The model under review builds one solid part; all positions refer to its coordinate system, in mm. A direction names the side the tool comes from. Coordinates: 2 decimals unless noted, no trailing zeros. Loops run counter-clockwise (first coordinate to the right, second up) from the corner with the lowest first, then second, coordinate; pieces in that order, holes last. Notation, with made-up numbers: (-4.75, 40) - (15.25, 40) arc R38 ccw to (15.25, 79) - close; hole circle Ø4 at (-37, 46.5). An arc over 180 degrees is marked (long way). One line per item, written item: value. Start each with the question number.
1. Insertion check: P1, Ø1.9, axis at x = 9, z = 8.5, coming from the -Y side; P2, Ø4, axis at x = 19.5, z = 2, coming from the +Y side; P3, Ø1.5, axis at x = 28, z = 8.5, coming from the +Y side. Each pin has a flat end and moves straight along its axis. Give the tip position at first contact, or say it passes through.
2. We need section B-B, the plane y = 3.5. Give the boundary of the cut face in (x, z), then the cut area to 3 significant figures.
3. We need section C-C, the plane x = 32. Give the boundary of the cut face in (y, z), then the cut area to 3 significant figures.
4. Mouldability with a two-part tool opening along X and no side actions: class faces 1 (the face through (29.115, -11.529, 7.395)), 2 (the face through (6.298, -2.507, 7.395)), 3 (the face through (14, 6, 15)), 4 (the face through (8.047, 13.33, 7.395)) as +X half, -X half, draft (parallel to the pull), parting line (faces both ways), or undercut.
5. For faces 5 (the face through (8.59, 13.79, 7.61)), 6 (the face through (16, 23, 7)), 7 (the face through (8, 23, 8)), 8 (the face through (5.8, 23.74, 7.53)), list the 3-axis set-ups (+Z, -Z, +X, -X, +Y, -Y) from which the entire face can be reached by the end or side of a thin tool; tool diameter is ignored.
6. To check wall thickness, follow line 1 (X direction, y = 0, z = 11); line 2 (X direction, y = -5, z = 13); line 3 (Y direction, x = 23, z = 2.5). State the ranges of each line that lie inside material, in increasing order.
from build123d import *

# Parameters (mm, degrees)
F1_DEPTH      = 15
F4_DEPTH      = 9.2
F4_DEPTH_BACK = 1
F7_DEPTH      = 1.5
F8_SIZE       = 1.49999
F9_R          = 5
F11_DEPTH     = 4
F12_T4_DEPTH  = 6.4753623201
F12_S5_R      = 22.299103121
F12_T6_DEPTH  = 5
F12_S8_R      = 5
F12_T9_DEPTH  = 5
F12_T13_DEPTH = 6.4753623415
F12_S15_R     = 5
F12_T16_DEPTH = 5
F12_S17_R     = 22.299103121
F12_T18_DEPTH = 5


# Not quite as in the source:
# - a fillet or chamfer that OpenCascade refuses, or shapes differently, is made with other operations: its cross-section is extruded or revolved along the edge and cut away or added
# - a fillet or chamfer is up to 0.001 mm smaller than in the source, because OpenCascade refuses the exact size


with BuildPart() as f1:
    # F0 (on Top) → F1 (new body)
    with BuildSketch(Plane.XY):
        with BuildLine():
            Line((37.0060966544, -19.4203102168), (21, -3.4142135624))
            Line((21, -3.4142135624), (21, 23))
            Line((21, 23), (8.9, 23))
            Line((8.9, 23), (8.0008047996, 12.8091210619))
            ThreePointArc((8.0008047996, 12.8091210619), (7.9975966714, 12.8026247244), (7.9908435011, 12.8))
            Line((7.9908435011, 12.8), (6.1708946074, 12.8))
            ThreePointArc((6.1708946074, 12.8), (3.6860466407, 11.9345702389), (2.2764293651, 9.7127652912))
            Line((2.2764293651, 9.7127652912), (-0.46875, -2))
            Line((-0.46875, -2), (-4.7960747033, -3))
            Line((-4.7960747033, -3), (17.7071067812, -2))
            Line((17.7071067812, -2), (17.7071067812, -4.7781745931))
            Line((17.7071067812, -4.7781745931), (34.6776695297, -21.7487373415))
            Line((34.6776695297, -21.7487373415), (37.0060966544, -19.4203102168))
        make_face()
    extrude(amount=F1_DEPTH)

    # F3 (on face) → F4 (cut, two sides)
    with BuildSketch(Plane(origin=(2.0824892704, 23.6015450644, 0), x_dir=(0.99612985, -0.0878938103, 0), z_dir=(-0.0878938103, -0.99612985, 0))) as f4_sk:
        with BuildLine():
            Line((6.8439980284, 15), (6.8439980284, 0))
            ThreePointArc((6.8439980284, 0), (8.1431011494, 7.5), (6.8439980284, 15))
        make_face()
    extrude(amount=F4_DEPTH, mode=Mode.SUBTRACT)
    extrude(f4_sk.sketch, amount=-F4_DEPTH_BACK, mode=Mode.SUBTRACT)

    # F6 (on offset) → F7 (join)
    with BuildSketch(Plane(origin=(0, 23, 0), x_dir=(-1, 0, 0), z_dir=(0, 1, 0))):
        with BuildLine():
            ThreePointArc((-7.0033527857, 9.4235612132), (-7.0960699027, 7.4999998768), (-7.0033527857, 5.5764385404))
            Line((-7.0033527857, 5.5764385404), (-5.4957957644, 5.5764385404))
            ThreePointArc((-5.4957957644, 5.5764385404), (-5.5960699027, 7.4999998768), (-5.4957957644, 9.4235612132))
            Line((-5.4957957644, 9.4235612132), (-7.0033527857, 9.4235612132))
        make_face()
        with BuildLine():
            Line((-14.0960699027, 7.4999998768), (-14.0960699027, 5.5764385404))
            Line((-14.0960699027, 5.5764385404), (-7.0033527857, 5.5764385404))
            ThreePointArc((-7.0033527857, 5.5764385404), (-7.0960699027, 7.4999998768), (-7.0033527857, 9.4235612132))
            Line((-7.0033527857, 9.4235612132), (-14.0960699027, 9.4235612132))
            Line((-14.0960699027, 9.4235612132), (-14.0960699027, 7.4999998768))
        make_face()
    extrude(amount=F7_DEPTH)

    # F8 (size 1.5 in the source; OpenCascade refuses exactly that, so slightly less here)
    f8_edges = [f1.edges().sort_by_distance(p)[0] for p in [
        (14.09607, 24.5, 7.5),
    ]]
    chamfer(f8_edges, length=F8_SIZE)

    # F9
    f9_edges = [f1.edges().sort_by_distance(p)[0] for p in [
        (12.59608, 24.5, 7.5),
    ]]
    fillet(f9_edges, radius=F9_R)

    # F10 (on face) → F11 (cut)
    with BuildSketch(Plane.XY.offset(9.4235612132)):
        Polygon((5.4957957644, 22), (6.5002299745, 22), (5.4957957644, 24.5), align=None)
    extrude(amount=-F11_DEPTH, mode=Mode.SUBTRACT)

    # F12: fillet of radius 1 on 3 edges, made by hand


with BuildPart() as f12_tool2:
    # F12_s3 → F12_t4 (new body)
    with BuildSketch(Plane.YZ.offset(7.6207075826)):
        with BuildLine():
            ThreePointArc((23, 10.4235612132), (23.2928932188, 9.716454432), (24, 9.4235612132))
            Line((24, 9.4235612132), (24, 9.4035612132))
            Line((24, 9.4035612132), (22.98, 9.4035612132))
            Line((22.98, 9.4035612132), (22.98, 10.4235612132))
            Line((22.98, 10.4235612132), (23, 10.4235612132))
        make_face()
    extrude(amount=F12_T4_DEPTH)

    # F12_s5 → F12_t6 (cut, symmetric)
    with BuildSketch(Plane(origin=(2.1446089712, 24.3055683406, 0), x_dir=(0, 0, 1), z_dir=(0.0878938103, 0.99612985, 0))):
        with Locations((7.5, -14.1560019716)):
            Circle(F12_S5_R)
    extrude(amount=F12_T6_DEPTH, both=True, mode=Mode.SUBTRACT)

    split(bisect_by=Plane.XZ.offset(-23), keep=Keep.BOTTOM)

    # F12_s8 → F12_t9 (intersect, symmetric)
    with BuildSketch(Plane.XY.offset(9.9)):
        with Locations((10.5250120908, 19.5)):
            Circle(F12_S8_R)
    extrude(amount=F12_T9_DEPTH, both=True, mode=Mode.INTERSECT)


with BuildPart() as f1_1:
    add(f1.part)

    # F12_t1: union F12_tool2
    add(f12_tool2.part)


with BuildPart() as f12_tool11:
    # F12_s12 → F12_t13 (new body)
    with BuildSketch(Plane.YZ.offset(14.0960699027)):
        with BuildLine():
            ThreePointArc((24, 5.5764385404), (23.2928932188, 5.2835453216), (23, 4.5764385404))
            Line((23, 4.5764385404), (22.98, 4.5764385404))
            Line((22.98, 4.5764385404), (22.98, 5.5964385404))
            Line((22.98, 5.5964385404), (24, 5.5964385404))
            Line((24, 5.5964385404), (24, 5.5764385404))
        make_face()
    extrude(amount=-F12_T13_DEPTH)

    split(bisect_by=Plane.XZ.offset(-23), keep=Keep.BOTTOM)

    # F12_s15 → F12_t16 (intersect, symmetric)
    with BuildSketch(Plane.XY.offset(5.1)):
        with Locations((10.5250120908, 19.5)):
            Circle(F12_S15_R)
    extrude(amount=F12_T16_DEPTH, both=True, mode=Mode.INTERSECT)

    # F12_s17 → F12_t18 (cut, symmetric)
    with BuildSketch(Plane(origin=(2.1446089712, 24.3055683406, 0), x_dir=(0, 0, 1), z_dir=(0.0878938103, 0.99612985, 0))):
        with Locations((7.5, -14.1560019716)):
            Circle(F12_S17_R)
    extrude(amount=F12_T18_DEPTH, both=True, mode=Mode.SUBTRACT)


with BuildPart() as f1_2:
    add(f1_1.part)

    # F12_t10: union F12_tool11
    add(f12_tool11.part)


solid = f1_2.part
Findings below:
1. P1: y = -2.43
1. P2: y = 23
1. P3: y = -9.66
2. outline: (0.82, 0) - (21, 0) - (21, 15) - (0.82, 15) - close
2. area: 303 mm2
3. outline: (-19.07, 0) - (-14.41, 0) - (-14.41, 15) - (-19.07, 15) - close
3. area: 69.9 mm2
4. face 1: +X half
4. face 2: undercut
4. face 3: draft
4. face 4: -X half
5. face 5: none
5. face 6: +X, +Y
5. face 7: -X
5. face 8: +Z, -Z, -X
6. line 1: 0 to 21
6. line 2: 17.93 to 22.59
6. line 3: -10.07 to -5.41
